Design review of the part built by this model. Coordinates are the model's own, in mm. A direction names the side the tool comes from. Coordinates: 2 decimals unless noted, no trailing zeros. Loops run counter-clockwise (first coordinate to the right, second up) from the corner with the lowest first, then second, coordinate; pieces in that order, holes last. Notation, with made-up numbers: (-31.75, -20) - (-4.75, -20) arc R20 ccw to (-4.75, -12) - close; hole circle Ø6 at (56, 44). An arc over 180 degrees is marked (long way). Use one line per item in the form item = value. Start each with the question number.
(1) Add section D-D (y = 0.5). State the section outline as (x, z) points, plus the area to 3 significant figures.
(2) Add section A-A (x = 8.25). State the section outline as (y, z) points, plus the area to 3 significant figures.
(3) For L1, parallel to Z at x = -1.75, y = 1.1; L2, parallel to X at y = 1.05, z = 21; L3, parallel to Z at x = 8.25, y = 0.4, list the stretches that pass through material, from the lowest coordinate up.
(4) Tool access review of faces 5 (the face through (-15.5, 1, 0)), 6 (the face through (11, 1, 22)), 7 (the face through (3, 1, -28)): name each direction out of +Z, -Z, +X, -X, +Y, -Y from which nothing blocks a thin tool from reaching the whole face with its end or side.
(5) Clearance check with flat-ended pins moving along their axes: pin 1 Ø4.5 at (x, z) = (0.544, -12.678) entering from +Y; pin 2 Ø0.8 at (y, z) = (0.5, 27) entering from +X; pin 3 Ø0.5 at (x, y) = (11, 0.5) entering from -Z. State where each tip first meets the part, or that it passes through.
(6) Add section B-B (x = 1). State the section outline as (y, z) points.
(7) The part is to be moulded in two halves that separate along Z. For faces 1 (the face through (3, 1, 28)), 2 (the face through (-9.051, 0.811, -16.096)), 3 (the face through (1, 1, 30)), 4 (the face through (11, 1, -22)), say which applies: pulls with the +Z half, pulls with the -Z half, needs draft (parallel to the pull), parting line crosses it, or undercut.
(8) Add section C-C (z = -12). State the section outline as (x, y) points.
Autodesk Inventor part; units mm, degrees
ref_plane "YZ Plane" through (0, 0, 0) normal (1, 0, 0) x (0, 1, 0)
ref_plane "XZ Plane" through (0, 0, 0) normal (0, 1, 0) x (-1, 0, 0)
ref_plane "XY Plane" through (0, 0, 0) normal (0, 0, 1) x (1, 0, 0)
sketch "Esquisse1" plane through (0, 0, 0) normal (0, 1, 0) x (-1, 0, 0)
  line L0 (15.5, -30) -> (-15.5, -30)
  line L1 (-15.5, -30) -> (-15.5, 30)
  line L2 (-15.5, 30) -> (15.5, 30)
  line L3 (15.5, 30) -> (15.5, -30)
  point P0 (0, 0)
  dimension "d0" = 31
  dimension "d1" = 60
  dimension "d2" = 30
  dimension "d3" = 15.5
extrude "Extrusion1" add sketch "Esquisse1" along normal blind 1.6
fillet "Congé1" radius 15 2 edges at (-15.5, 0.8, -30) (-15.5, 0.8, 30)
sketch "Esquisse2" plane through (0, 1.6, 0) normal (0, 1, 0) x (1, 0, 0)
  circle A0 centre (7, 26) radius 4
  circle A1 centre (7, -26) radius 4
  line L0 (-0.5, -30) -> (15.5, -30)
  line L1 (3, 26) -> (3, 30)
  line L2 (15.5, 30) -> (-0.5, 30)
  line L3 (7, 30) -> (3, 30)
  line L4 (7, 30) -> (15.5, 30)
  line L5 (15.5, 30) -> (15.5, 22)
  line L6 (15.5, -30) -> (15.5, 30)
  line L7 (15.5, 22) -> (7, 22)
  line L8 (7, -22) -> (15.5, -22)
  line L9 (15.5, -22) -> (15.5, -30)
  line L10 (15.5, -30) -> (7, -30)
  line L11 (3, -26) -> (3, -30)
  line L12 (3, -30) -> (7, -30)
  point P0 (0, 0)
  dimension "d7" = 8
  dimension "d8" = 7
  dimension "d9" = 7
  dimension "d10" = 26
  dimension "d11" = 26
extrude "Extrusion3" cut sketch "Esquisse2" against normal through all
sketch "Esquisse3" plane through (0, 1.6, 0) normal (0, 1, 0) x (1, 0, 0)
  circle A0 centre (-9.75, 15) radius 1.3
  circle A1 centre (-1.75, -26) radius 1.3
  circle A2 centre (8.25, 18) radius 1.3
  line L0 (-15.5, 15) -> (-15.5, -15)
  circle A3 centre (2.689, -19.678) radius 2.5
  circle A4 centre (0.544, 12.678) radius 2.5
  point P0 (0, 0)
  dimension "d19" = 2.6
  dimension "d20" = 2.6
  dimension "d21" = 2.6
  dimension "d23" = 13.75
  dimension "d24" = 15
  dimension "d25" = 5.75
  dimension "d26" = 18
  dimension "d27" = 8.25
  dimension "d30" = 15.5
  dimension "d31" = 11
  dimension "d32" = 5
  dimension "d33" = 5
  dimension "d34" = 34.678
  dimension "d35" = 2.322
  dimension "d36" = 18.189
  dimension "d37" = 16.044
extrude "Extrusion4" cut sketch "Esquisse3" against normal blind 18.189
equation "\"d20\" = d19"
equation "\"d21\" = d19"
equation "\"d33\" = d32"
equation "\"d28\" = d36"
properties part number "PCB Droit" material "Nylon, disulfure de molybdène"
Computed values:
q1.outline = (-15.5, -15) arc R15 ccw to (-0.5, -30) - (3, -30) - (3, -26) arc R4 cw to (7, -22) - (15.5, -22) - (15.5, 22) - (7, 22) arc R4 cw to (3, 26) - (3, 30) - (-0.5, 30) arc R15 ccw to (-15.5, 15) - close; hole circle Ø2.6 at (-9.75, -15); hole circle Ø2.6 at (-1.75, 26); hole circle Ø5 at (0.54, -12.68); hole circle Ø5 at (2.69, 19.68); hole circle Ø2.6 at (8.25, -18)
q1.area = 1,520 mm^2
q2.outline = (0, -22) - (1.6, -22) - (1.6, -19.3) - (0, -19.3) - close; (0, -16.7) - (1.6, -16.7) - (1.6, 22) - (0, 22) - close
q2.area = 66.2 mm^2
q3.L1 = -29.95 to -13.67, -11.68 to 24.7, 27.3 to 29.95
q3.L2 = -14.25 to 0.57, 4.81 to 15.5
q3.L3 = -22 to -19.3, -16.7 to 22
q4.face_5 = +Z, -Z, -X, +Y, -Y
q4.face_6 = +Z, +X, +Y, -Y
q4.face_7 = -Z, +X, +Y, -Y
q5.pin_1 = through
q5.pin_2 = 3
q5.pin_3 = -22
q6.outline = (0, -30) - (1.6, -30) - (1.6, -15.14) - (0, -15.14) - close; (0, -10.22) - (1.6, -10.22) - (1.6, 17.83) - (0, 17.83) - close; (0, 21.52) - (1.6, 21.52) - (1.6, 30) - (0, 30) - close
q7.face_1 = needs draft
q7.face_2 = undercut
q7.face_3 = pulls with the +Z half
q7.face_4 = pulls with the -Z half
q8.outline = (-15.5, 0) - (-1.86, 0) - (-1.86, 1.6) - (-15.5, 1.6) - close; (2.95, 0) - (15.5, 0) - (15.5, 1.6) - (2.95, 1.6) - close
